```python
from build123d import *

# Parameters (mm, degrees)
SKETCH1_W           = 20.735936364
SKETCH1_H           = 3.175
BOSS_EXTRUDE1_DEPTH = 6.35
SKETCH2_W           = 82.651107169
SKETCH2_H           = 6.52720724
SKETCH2_W_2         = 76.969823319
SKETCH2_H_2         = 6.604
CUT_EXTRUDE1_DEPTH  = 7.35
SKETCH6_W           = 206.502
SKETCH6_H           = 3.711703494
SKETCH6_H_2         = 2.816288331
BOSS_EXTRUDE3_DEPTH = 25.4
BOSS_EXTRUDE5_DEPTH = 136.779


with BuildPart() as part:
    # Sketch1 → Boss-Extrude1 (new body)
    with BuildSketch(Plane(origin=(0, 0, 0), x_dir=(0, 0, -1), z_dir=(1, 0, 0))):
        Polygon((-123.525645009, 81.218983384), (-123.525645009, -25.082949612), (-102.22101814, -26.860004783), (-104.557017494, 0), (-79.646789796, 17.686261666), (-41.094549164, 17.686261666), (-13.779824281, -3.641289166), (-17.947471695, -33.889404663), (-12.561862574, -34.338627482), (90.228248196, -18.303088648), (90.228248196, 91.281577209), (0, 117.577378193), (-20.735936364, 117.577378193), align=None)
        Polygon((5.201841666, 40.001048477), (77.528248196, 55.056292197), (77.528248196, 85.830387495), (5.201841666, 105.015188817), align=None, mode=Mode.SUBTRACT)
        Polygon((-79.646789796, 84.224142025), (-79.646789796, 48.574048336), (0, 40.007327233), (0, 105.015188817), (-20.735936364, 105.015188817), align=None, mode=Mode.SUBTRACT)
        Polygon((-86.090479579, 81.218983384), (-86.090479579, 50.197772081), (-114.759972161, 55.666680192), (-114.759972161, 71.350976637), align=None, mode=Mode.SUBTRACT)
        with Locations((-10.367968182, 112.814878193)):
            Rectangle(SKETCH1_W, SKETCH1_H, mode=Mode.SUBTRACT)
    extrude(amount=BOSS_EXTRUDE1_DEPTH)

    # Sketch2 → Cut-Extrude1 (cut, through all)
    with BuildSketch(Plane(origin=(6.35, 0, 0), x_dir=(0, 0, -1), z_dir=(1, 0, 0))):
        with Locations((117.850801407, 29.125465717)):
            Rectangle(SKETCH2_W, SKETCH2_H)
        with Locations((-85.04073335, 29.163862097)):
            Rectangle(SKETCH2_W_2, SKETCH2_H_2)
    extrude(amount=-CUT_EXTRUDE1_DEPTH, mode=Mode.SUBTRACT)

    # Sketch6 → Boss-Extrude3 (add)
    with BuildSketch(Plane.ZY):
        with Locations((20.274645009, 34.244921084)):
            Rectangle(SKETCH6_W, SKETCH6_H)
        with Locations((20.274645009, 24.453717932)):
            Rectangle(SKETCH6_W, SKETCH6_H_2)
    extrude(amount=BOSS_EXTRUDE3_DEPTH)

    # Sketch8 → Boss-Extrude5 (add)
    with BuildSketch(Plane.ZY):
        Polygon((0, 117.577378193), (-83.878248196, 93.218298083), (-90.228248196, 91.281577209), (-90.228248196, 32.389069337), (-83.878248196, 32.389069337), (-83.878248196, 86.868298083), (-9.525197863, 108.461165703), (29.097772116, 108.270149457), (123.542635704, 74.868983384), (123.525645009, 81.218983384), (20.735936364, 117.577378193), (20.752927059, 113.344232588), (26.228286967, 113.344232588), (26.228286967, 111.139694939), (20.752927059, 111.139694939), (0.016990695, 111.139694939), (-7.377605414, 111.139694939), (-7.377605414, 113.344232588), (0.011172356, 113.344232588), align=None)
    extrude(amount=BOSS_EXTRUDE5_DEPTH)


solid = part.part
```
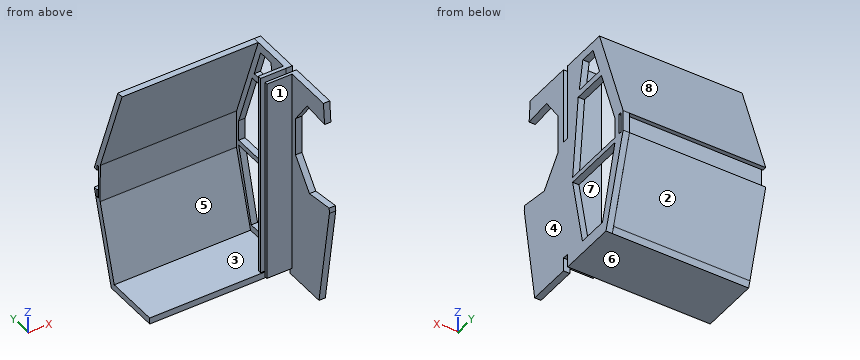
Geometry check sheet. Reference: the model listing, model coordinates, mm. Face numbers are marked on the shaded views. A direction names the side the tool comes from. Give positions to 0.01 mm unless a question says otherwise; leave off trailing zeros. Loops run counter-clockwise (first coordinate to the right, second up) from the corner with the lowest first, then second, coordinate; pieces in that order, holes last. Notation, with made-up numbers: (66, 44.5) - (81, 44.5) arc R29 ccw to (81, 66.5) - close; hole circle Ø7 at (77, 20.25). An arc over 180 degrees is marked (long way). Use CSV: the item, a comma, the result in double quotes. Start each with the question number.
Q1. Release check for a two-part mould opening along Y. For the marked faces 6, 7 and 8 record: +Y half, -Y half, draft (parallel to the pull), parting line (faces both ways), or undercut.
Q2. Access from +Z, -Z, +X, -X, +Y, -Y to the whole of each face (thin tool, end or side, straight path). Record for the marked faces 1, 2, 3, 4 and 5.
Q3. Section check A-A, the plane x = -2.5. Record the cut outline in (y, z), and give its area (3 significant figures).
Q4. Section check B-B, the plane y = 67.5. Record the cut outline in (x, z), and give its area (3 significant figures).
Q5. Section check C-C, the plane y = 7.5. Record the cut outline in (x, z).
Q6. Scan lines: probe 1 along Y at (x, z) = (-5, 85); probe 2 along Z at (x, y) = (-66, 73.5); probe 3 along Y at (x, z) = (-23, -79.5). Record each from-to range of solid material in increasing order. Write a range as from..to.
Q7. Section check D-D, the plane z = 8.5. Record the cut outline in (x, y), and give its area (3 significant figures).
Q8. Go/stop test with flat-tipped pins: pin 1 Ø1.6 at (x, z) = (-39.5, 22.5) entering from -Y; pin 2 Ø3 at (x, z) = (4.5, 66.5) entering from -Y; pin 3 Ø4 at (x, z) = (-52, 18) entering from +Y. Record where each tip stops, or that it passes through.
Findings below:
1,face 6,"draft"
1,face 7,"undercut"
1,face 8,"+Y half"
2,face 1,"+Z, -Z, -X, -Y"
2,face 2,"-Z, +X, -X, +Y"
2,face 3,"-X, -Y"
2,face 4,"+Z, -Z, +X, +Y, -Y"
2,face 5,"-X"
3,outline,"(23.05, -82.98) - (25.86, -82.98) - (25.86, 123.53) - (23.05, 123.53) - close; (32.39, -90.23) - (91.28, -90.23) - (93.22, -83.88) - (117.58, 0) - (113.34, 0.01) - (113.34, -7.38) - (111.14, -7.38) - (111.14, 26.23) - (113.34, 26.23) - (113.34, 20.75) - (117.58, 20.74) - (81.22, 123.53) - (74.87, 123.54) - (108.27, 29.1) - (108.46, -9.53) - (86.87, -83.88) - (32.39, -83.88) - close; (32.39, -82.98) - (36.1, -82.98) - (36.1, 123.53) - (32.39, 123.53) - close"
3,area,"2,970 mm^2"
4,outline,"(-136.78, -90.23) - (6.35, -90.23) - (6.35, -77.53) - (0, -77.53) - (0, -83.88) - (-136.78, -83.88) - close; (0, -5.2) - (6.35, -5.2) - (6.35, 0) - (0, 0) - close; (0, 79.65) - (6.35, 79.65) - (6.35, 86.09) - (0, 86.09) - close; (0, 114.76) - (6.35, 114.76) - (6.35, 123.53) - (0, 123.53) - close"
4,area,"1,080 mm^2"
5,outline,"(0, -90.23) - (6.35, -90.23) - (6.35, 28.05) - (0, 28.05) - close; (0, 93.99) - (6.35, 93.99) - (6.35, 123.53) - (0, 123.53) - close"
6,probe 1,"y = 23.05..25.86, 32.39..36.1, 88.5..94.85"
6,probe 2,"z = -90.23..-83.88"
6,probe 3,"y = 23.05..25.86, 32.39..36.1, 88.14..94.49"
7,outline,"(-136.78, 108.37) - (0, 108.37) - (0, 105.02) - (6.35, 105.02) - (6.35, 111.23) - (0, 111.23) - (0, 111.14) - (-136.78, 111.14) - close; (-25.4, 23.05) - (0, 23.05) - (0, -33.7) - (6.35, -33.7) - (6.35, 40.92) - (0, 40.92) - (0, 36.1) - (-25.4, 36.1) - (-25.4, 32.39) - (0, 32.39) - (0, 25.86) - (-25.4, 25.86) - close; (0, 114.4) - (6.35, 114.4) - (6.35, 117.58) - (0, 117.58) - close"
7,area,"1,080 mm^2"
8,pin 1,"stops at y = 108.3"
8,pin 2,"stops at y = 17.69"
8,pin 3,"stops at y = 111.14"
